Solid Edge part; units mm, degrees
sketch "Sketch1" plane through (0, 0, 0) normal (0, 1, 0) x (-1, 0, 0)
  circle A0 centre (16.756, -24.8845) radius 2.25
  circle A1 centre (27.4161, 12.1803) radius 2.25
  circle A2 centre (-7.2345, 29.1146) radius 2.25
  circle A3 centre (-21.5968, -20.8226) radius 2.25
  circle A4 centre (0, -32) radius 2.8
  circle A5 centre (0, 32) radius 2.8
  circle A6 centre (0, 0) radius 39
  circle A7 centre (-32, 0) radius 2.8
  circle A8 centre (32, 0) radius 2.8
  circle A9 centre (-24.2565, 17.6529) radius 2.25
  circle A10 centre (13.1726, 26.9533) radius 2.25
  circle A11 centre (28.8313, -8.2921) radius 2.25
  circle A12 centre (0, 0) radius 17.5
extrude "Protrusion1" add sketch "Sketch1" along normal blind 15
sketch "Sketch2" plane through (0, 15, 0) normal (0, 1, 0) x (-1, 0, 0)
  circle A0 centre (27.4161, 12.1803) radius 2.25
  circle A1 centre (32, 0) radius 2.8
  circle A2 centre (13.1726, 26.9533) radius 2.25
  circle A3 centre (16.756, -24.8845) radius 2.25
  circle A4 centre (28.8313, -8.2921) radius 2.25
  circle A5 centre (0, -32) radius 2.8
  arc A6 (4.5655, 16.894) -> (-4.4574, -16.9228) centre (0, 0) cw
  line L0 (-4.4574, -16.9228) -> (-10, -37.6962)
  arc A7 (10.1123, 37.6662) -> (-10, -37.6962) centre (0, 0) cw
  line L1 (10.1123, 37.6662) -> (10, 37.262)
  line L2 (10, 37.262) -> (4.5655, 16.894)
extrude "ExtrudedCutout_1" cut sketch "Sketch2" along normal mid plane 476
sketch "Sketch3" plane through (14.4439, 0, 0.6519) normal (0, -1, 0) x (-0.2578, 0, 0.9662)
  line L0 (51.6742, 10.1797) -> (37.8149, -3.6369)
  line L1 (37.8149, -3.6369) -> (41.6742, 14.1797)
  line L2 (41.6742, 14.1797) -> (51.6742, 14.1797)
  line L3 (51.6742, 14.1797) -> (51.6742, 10.1797)
extrude "Protrusion2" add sketch "Sketch3" against normal up to vertex (15 mm away)
sketch "Sketch4" plane through (-7.4783, 7.5, 43.3268) normal (-0.9662, 0, -0.2578) x (-0.2578, 0, 0.9662)
  circle A0 centre (0, 0) radius 2.25
extrude "ExtrudedCutout_2" cut sketch "Sketch4" along normal mid plane 49.6
sketch "Sketch5" plane through (-7.4783, 7.5, 43.3268) normal (-0.9662, 0, -0.2578) x (-0.2578, 0, 0.9662)
  circle A0 centre (0, 0) radius 4
extrude "ExtrudedCutout_3" cut sketch "Sketch5" against normal blind 13.9
mirror "Mirror1" about plane through (1.8783, 7.5, 0.5012) normal (-0.2578, 0, 0.9662) of "Protrusion2", "ExtrudedCutout_2", "ExtrudedCutout_3"
sketch "Sketch6" plane through (0, 0, 0) normal (0, 1, 0) x (-1, 0, 0)
  arc A0 (-10, -37.6962) -> (-26.1113, -28.9689) centre (0, 0) cw
  arc A1 (-26.1113, -28.9689) -> (-8.2093, 38.1262) centre (0, 0) cw
  arc A2 (-8.2093, 38.1262) -> (10.1081, 37.6673) centre (0, 0) cw
  arc A3 (10.1081, 37.6673) -> (10.1123, 37.6662) centre (0, 0) cw
  line L0 (10.1123, 37.6662) -> (10, 37.262)
  line L1 (10, 37.262) -> (4.5655, 16.894)
  arc A4 (-4.4574, -16.9228) -> (4.5655, 16.894) centre (0, 0) cw
  line L2 (-4.4574, -16.9228) -> (-10, -37.6962)
extrude "Protrusion3" add sketch "Sketch6" along normal up to vertex (15 mm away)
sketch "Sketch7" plane through (13.211, 15, 0.5012) normal (0, 1, 0) x (0.2578, 0, -0.9662)
  circle A0 centre (-22.6453, -9.7111) radius 2.25
  circle A1 centre (-3.5007, -17.1007) radius 2.25
  circle A2 centre (15.9148, -10.4557) radius 2.25
  circle A3 centre (26.5166, 7.1148) radius 2.25
extrude "ExtrudedCutout_5" cut sketch "Sketch7" against normal blind 56.1
sketch "Sketch8" plane through (0, 0, 0) normal (0, 1, 0) x (-1, 0, 0)
  circle A0 centre (-32, 0) radius 2.8
extrude "ExtrudedCutout_6" cut sketch "Sketch8" along normal blind 110.3
sketch "Sketch9" plane through (13.211, 0, 0.5012) normal (0, -1, 0) x (0.2578, 0, -0.9662)
  line L0 (-25.5718, 12.135) -> (-26.2077, 8.3886)
  line L1 (-26.2077, 8.3886) -> (-23.2811, 5.9647)
  line L2 (-23.2811, 5.9647) -> (-19.7187, 7.2872)
  line L3 (-19.7187, 7.2872) -> (-19.0828, 11.0336)
  line L4 (-19.0828, 11.0336) -> (-22.0094, 13.4575)
  line L5 (-22.0094, 13.4575) -> (-25.5718, 12.135)
  line L6 (-6.6629, 19.208) -> (-6.9068, 15.4159)
  line L7 (-6.9068, 15.4159) -> (-3.7446, 13.3086)
  line L8 (-3.7446, 13.3086) -> (-0.3386, 14.9934)
  line L9 (-0.3386, 14.9934) -> (-0.0947, 18.7856)
  line L10 (-0.0947, 18.7856) -> (-3.2568, 20.8929)
  line L11 (-3.2568, 20.8929) -> (-6.6629, 19.208)
  line L12 (17.9517, 13.6636) -> (14.1551, 13.8237)
  line L13 (14.1551, 13.8237) -> (12.1182, 10.6157)
  line L14 (12.1182, 10.6157) -> (13.8779, 7.2477)
  line L15 (13.8779, 7.2477) -> (17.6745, 7.0877)
  line L16 (17.6745, 7.0877) -> (19.7114, 10.2956)
  line L17 (19.7114, 10.2956) -> (17.9517, 13.6636)
extrude "ExtrudedCutout_7" cut sketch "Sketch9" against normal blind 3
sketch "Sketch10" plane through (13.211, 0, 0.5012) normal (0, -1, 0) x (0.2578, 0, -0.9662)
  line L0 (22.7166, -7.1148) -> (24.6166, -10.4057)
  line L1 (24.6166, -10.4057) -> (28.4166, -10.4057)
  line L2 (28.4166, -10.4057) -> (30.3166, -7.1148)
  line L3 (30.3166, -7.1148) -> (28.4166, -3.8239)
  line L4 (28.4166, -3.8239) -> (24.6166, -3.8239)
  line L5 (24.6166, -3.8239) -> (22.7166, -7.1148)
extrude "ExtrudedCutout_8" cut sketch "Sketch10" against normal blind 3
Here's how the part is built. I have some questions about the finished solid (model axes, mm). A direction names the side the tool comes from. Round coordinates to 2 decimals unless told otherwise and drop trailing zeros. Order: outer loops, then holes, each group sorted by start corner. A loop starts at its lowest first (then second) coordinate and runs counter-clockwise, first axis right, second up. Notation, with made-up numbers: M -35.75,50.25 L 21.25,50.25 A8 ccw 21.25,62.25 Z; hole C -30.75,28.5 d2. An arc over 180 degrees is marked long. Use CSV: the item, a comma, the result in double quotes.
1) I want a section at A-A (z = 0). List the corners of the cut face in (x, y) for me, then the cut area to 4 significant figures.
Taken from the geometry:
outline,"M 17.5,0 L 29.2,0 L 29.2,15 L 17.5,15 Z; M 34.8,0 L 39,0 L 39,15 L 34.8,15 Z"
area,"238.5 mm^2"
2) I need wall thicknesses on line 1 along Z through (x, y) = (28, 3.25); line 2 along Z through (x, y) = (30.5, 6.75); line 3 along Y through (x, z) = (15.5, -25). Which ranges of each line are inside material? Lowest first, please. Write a range as [from, to].
Taken from the geometry:
line 1,"[-27.15, -14.35], [-10.01, 6.2], [10.38, 27.15]"
line 2,"[-24.31, -2.36], [2.36, 6.78], [9.8, 24.31]"
line 3,"[3, 15]"
3) If we mould it in two halves opening along Y, with no side actions, what happens to faces 3 (the flat face through (19, 15, 10)), 4 (the cylindrical face through (37.832, 7.395, 9.474)), 5 (the cylindrical face through (17.323, 7.324, -36.564)), 6 (the cylindrical face through (12.77, 9.02, -40.2))? For each: pulls with the +Y half, pulls with the -Y half, needs draft (parallel to the pull), parting line crosses it, or undercut.
Taken from the geometry:
face 3,"pulls with the +Y half"
face 4,"needs draft"
face 5,"undercut"
face 6,"undercut"
4) On a 3-axis mill with a long thin cutter (end or side, diameter ignored), from which of +Z, -Z, +X, -X, +Y, -Y can I reach the whole of each face in a straight line? I mean faces 1 (the cylindrical face through (18.124, 9.084, 23.099)), 2 (the flat face through (17.034, 1.479, 21.605)). Say none if no direction works.
Taken from the geometry:
face 1,"+Y, -Y"
face 2,"-Y"
5) I'm going to push flat-ended pins straight in: P1, Ø8, axis at y = 10, z = 11, coming from the +X side; P2, Ø2, axis at x = 27, z = -14, coming from the -Y side; P3, Ø1.5, axis at x = 20, y = 1.5, coming from the +Z side; P4, Ø2.5, axis at x = 16.76, z = 24.88, coming from the +Y side. Where does each tip first touch, or does it pass through?
Taken from the geometry:
P1,"x = 38.37"
P2,"y = 3"
P3,"z = 33.92"
P4,"through"
6) I want a section at C-C (y = 1.25). Count the separate pieces of the cut face and the enclosed holes in it, then the cut area to 3 significant figures.
Taken from the geometry:
separate pieces,"1"
enclosed holes,"5"
area,"1,940 mm^2"
7) I want a section at B-B (x = 6). List the corners of the cut face in (y, z) for me.
Taken from the geometry:
outline,"M 0,-22.7 L 15,-22.7 L 15,-16.44 L 0,-16.44 Z; M 0,16.44 L 15,16.44 L 15,39.41 L 0,39.41 Z"
